Source: CAD feature listing. Evaluate the final solid. Frame: model axes, mm. Coordinates: 2 decimals unless noted, no trailing zeros. Write each loop counter-clockwise with the first axis right and the second up, starting at its lowest first coordinate (ties: lowest second). Pieces come first, ordered by that corner, then holes. Notation, with made-up numbers: (11.25, 49) - (65.25, 49) arc R26 cw to (65.25, 70) - close; hole circle Ø3 at (-23, 60). An arc over 180 degrees is marked (long way). One line per question, with ' | ' between items.
from build123d import *

# Parameters (mm, degrees)
SKETCH_1_R          = 7.5
EXTRUDE_1_DEPTH     = 92
SKETCH_2_R          = 6
CUT_EXTRUDE_1_DEPTH = 34.59
CUT_EXTRUDE_START   = -34.59
SKETCH_3_R          = 6
CUT_EXTRUDE_2_DEPTH = 34.59


with BuildPart() as part:
    # 스케치1 → 보스-돌출1 (new, symmetric)
    with BuildSketch(Plane.XY):
        Circle(SKETCH_1_R)
    extrude(amount=EXTRUDE_1_DEPTH, both=True)

    # 스케치2 → 컷-돌출1 (cut)
    with BuildSketch(Plane.XY.offset(92)):
        Circle(SKETCH_2_R)
    extrude(amount=-CUT_EXTRUDE_1_DEPTH, mode=Mode.SUBTRACT)

    # 스케치3 → 컷-돌출2 (cut)
    with BuildSketch(Plane(origin=(0, 0, -92), x_dir=(-1, 0, 0), z_dir=(0, 0, -1)).offset(CUT_EXTRUDE_START)):
        with Locations(Location((0, 0, 0), (0, 0, 180))):
            Circle(SKETCH_3_R)
    extrude(amount=CUT_EXTRUDE_2_DEPTH, mode=Mode.SUBTRACT)


solid = part.part
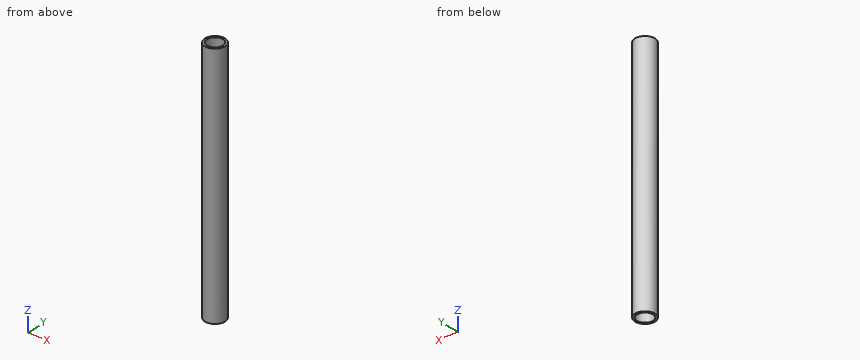
Item 1: Ray query, line 1 along Y through (x, z) = (0, -71); line 2 along X through (y, z) = (0.25, 67.5); line 3 along Z through (x, y) = (-3.75, -2.25). Return the intervals inside material, ascending. Write a range as [from, to].
Check sheet entries:
line 1: [-7.5, -6], [6, 7.5] | line 2: [-7.5, -5.99], [5.99, 7.5] | line 3: [-57.41, 57.41]
Item 2: Cut plane D-D on z = 42. Return loops of the section in (x, y), and give its area (3 significant figures).
Check sheet entries:
outline: circle Ø15 at (0, 0) | area: 177 mm²
Item 3: Cut plane C-C on z = 71.5. Return loops of the section in (x, y).
Check sheet entries:
outline: circle Ø15 at (0, 0); hole circle Ø12 at (0, 0)
Item 4: Pin query (flat end, axial travel): pin 1 Ø3 at (y, z) = (5.5, 44) entering from +X; pin 2 Ø6 at (x, y) = (-2, -3.5) entering from -Z; pin 3 Ø4 at (x, z) = (-4.5, 69) entering from -Y; pin 4 Ø1 at (y, z) = (2, 5.5) entering from +X. Return the tip coordinate at first contact, or that it passes through.
Check sheet entries:
pin 1: x = 6.34 | pin 2: z = -92 | pin 3: y = -7.07 | pin 4: x = 7.35
Item 5: Cut plane A-A on x = 0. Return loops of the section in (y, z).
Check sheet entries:
outline: (-7.5, -92) - (-6, -92) - (-6, -57.41) - (6, -57.41) - (6, -92) - (7.5, -92) - (7.5, 92) - (6, 92) - (6, 57.41) - (-6, 57.41) - (-6, 92) - (-7.5, 92) - close
